from build123d import *

# Parameters (mm, degrees)
SKETCH1_W           = 154
SKETCH1_H           = 27
BOSS_EXTRUDE1_DEPTH = 0.1
CUT_EXTRUDE1_DEPTH  = 79.174548288


with BuildPart() as part:
    # Sketch1 → Boss-Extrude1 (new body)
    with BuildSketch(Plane(origin=(0, 0, 0), x_dir=(1, 0, 0), z_dir=(0, 1, 0))):
        Rectangle(SKETCH1_W, SKETCH1_H)
    extrude(amount=BOSS_EXTRUDE1_DEPTH)

    # Sketch2 → Cut-Extrude1 (cut, through all)
    with BuildSketch(Plane(origin=(0, 0.1, 0), x_dir=(1, 0, 0), z_dir=(0, 1, 0))):
        with BuildLine():
            Line((2.4, 5.00499584), (2.4, -1.00499584))
            ThreePointArc((2.4, -1.00499584), (15.3, 2), (2.4, 5.00499584))
        make_face()
        with BuildLine():
            Line((38.4, 5.00499584), (38.4, -1.00499584))
            ThreePointArc((38.4, -1.00499584), (51.3, 2), (38.4, 5.00499584))
        make_face()
        with BuildLine():
            Line((-33.6, 5.00499584), (-33.6, -1.00499584))
            ThreePointArc((-33.6, -1.00499584), (-20.7, 2), (-33.6, 5.00499584))
        make_face()
        with BuildLine():
            Line((-62.6, 5.00499584), (-62.6, -1.00499584))
            ThreePointArc((-62.6, -1.00499584), (-49.7, 2), (-62.6, 5.00499584))
        make_face()
    extrude(amount=-CUT_EXTRUDE1_DEPTH, mode=Mode.SUBTRACT)


solid = part.part
For this review, take the finished solid that the model builds, in its own axes (mm). Give positions to 0.01 mm unless a question says otherwise; leave off trailing zeros. Loops run counter-clockwise (first coordinate to the right, second up) from the corner with the lowest first, then second, coordinate; pieces in that order, holes last. Notation, with made-up numbers: M 61.5,-14 L 90.5,-14 A7 cw 90.5,-5 Z; hole C 68.5,-9.5 d3. An arc over 180 degrees is marked long. Put each result on its own line as item: value. Start each with the question number.
(1) Add section C-C, the plane y = 0.05. Write out the cut boundary in (x, z) (3 decimals), then the cut area to 3 significant figures.
(2) Add section A-A, the plane x = 8.5. Write out the cut boundary in (y, z), then the cut area to 3 significant figures.
(3) Add section B-B, the plane z = -2. Write out the cut boundary in (x, y), then the cut area to 3 significant figures.
(4) For pin 1 (15.5 mm diameter, centred on x = -27.5, z = -2, fed in from -Y), flat-tipped, find the tip position at first contact; note if it passes through.
(5) Wall thickness on L1, parallel to X at y = 0.05, z = -2; L2, parallel to X at y = 0.05, z = -8.25: over which ranges is each line inside the solid? List them lowest first.
Result:
1. outline: M -77,-13.5 L 77,-13.5 L 77,13.5 L -77,13.5 Z; hole M -62.6,-5.005 A6.8 ccw long -62.6,1.005 Z; hole M -33.6,-5.005 A6.8 ccw long -33.6,1.005 Z; hole M 2.4,-5.005 A6.8 ccw long 2.4,1.005 Z; hole M 38.4,-5.005 A6.8 ccw long 38.4,1.005 Z
1. area: 3,590 mm^2
2. outline: M 0,-13.5 L 0.1,-13.5 L 0.1,-8.8 L 0,-8.8 Z; M 0,4.8 L 0.1,4.8 L 0.1,13.5 L 0,13.5 Z
2. area: 1.34 mm^2
3. outline: M -77,0 L -62.6,0 L -62.6,0.1 L -77,0.1 Z; M -49.7,0 L -33.6,0 L -33.6,0.1 L -49.7,0.1 Z; M -20.7,0 L 2.4,0 L 2.4,0.1 L -20.7,0.1 Z; M 15.3,0 L 38.4,0 L 38.4,0.1 L 15.3,0.1 Z; M 51.3,0 L 77,0 L 77,0.1 L 51.3,0.1 Z
3. area: 10.2 mm^2
4. pin 1: stops at y = 0
5. L1: x = -77 to -62.6, -49.7 to -33.6, -20.7 to 2.4, 15.3 to 38.4, 51.3 to 77
5. L2: x = -77 to -59.18, -53.82 to -30.18, -24.82 to 5.82, 11.18 to 41.82, 47.18 to 77
